Verification items for this drawing (mm, ordinates from the low corner). Coordinates: 2 decimals unless noted, no trailing zeros. Order: outer loops, then holes, each group sorted by start corner. A loop starts at its lowest first (then second) coordinate and runs counter-clockwise, first axis right, second up. Notation, with made-up numbers: M 1,-32.5 L 54,-32.5 A27 cw 54,-4.5 Z; hole C 8.5,18.25 d4. An arc over 180 degrees is marked long. One line per item, written item: value. Start each with the question number.
1) Sectioned sample at A-A, the plane x = 54.5. Enter the section's corners in (y, z), then the cut area to 3 significant figures.
2) Sectioned sample at D-D, the plane z = 24. Enter the section's corners in (x, y), then the cut area to 3 significant figures.
3) Sectioned sample at C-C, the plane z = 85.5. Enter the section's corners in (x, y).
4) Thickness scan on L1, parallel to X at y = 3.7, z = 20; L2, parallel to Z at x = 54.5, y = 3.35; L3, parallel to X at y = 2, z = 48. Record the ranges inside material, lowest first. Write a range as from..to.
5) Go/stop test with a flat-tipped pin: P1, Ø1, axis at x = 35, y = 2, coming from the +Z side. Record where the tip stops, or that it passes through.
6) Sectioned sample at B-B, the plane y = 3.65. State how many separate pieces and enclosed holes the cut face has, then the cut area to 3 significant figures.
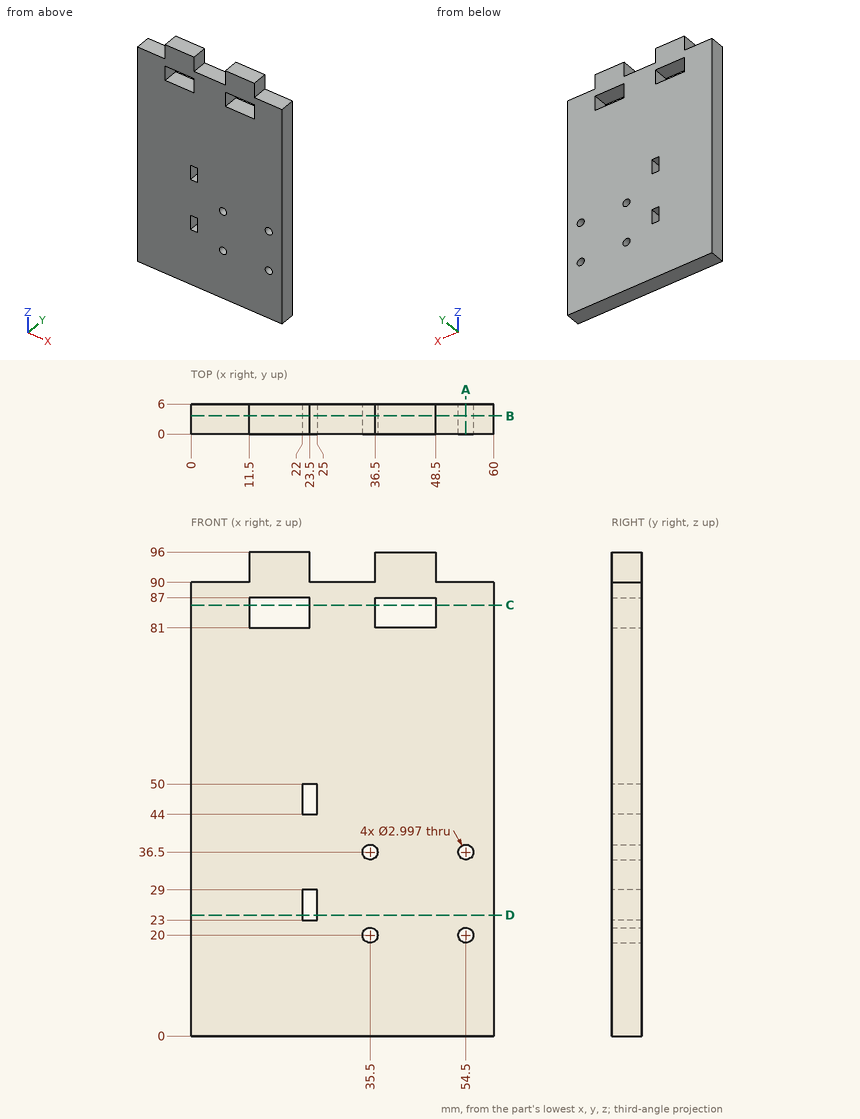
Final values:
1. outline: M 0,0 L 6,0 L 6,18.5 L 0,18.5 Z; M 0,21.5 L 6,21.5 L 6,35 L 0,35 Z; M 0,38 L 6,38 L 6,90 L 0,90 Z
1. area: 504 mm^2
2. outline: M 0,0 L 22,0 L 22,6 L 0,6 Z; M 25,0 L 60,0 L 60,6 L 25,6 Z
2. area: 342 mm^2
3. outline: M 0,0 L 11.5,0 L 11.5,6 L 0,6 Z; M 23.5,0 L 36.5,0 L 36.5,6 L 23.5,6 Z; M 48.5,0 L 60,0 L 60,6 L 48.5,6 Z
4. L1: x = 0..34, 37..53, 56..60
4. L2: z = 0..18.5, 21.5..35, 38..90
4. L3: x = 0..22, 25..60
5. P1: stops at z = 90
6. separate pieces: 1
6. enclosed holes: 8
6. area: 5,340 mm^2
